Build history of the part. All positions in model axes, mm. Round coordinates to 2 decimals unless told otherwise and drop trailing zeros. Write each loop counter-clockwise with the first axis right and the second up, starting at its lowest first coordinate (ties: lowest second). Pieces come first, ordered by that corner, then holes.
Item 1: Band-saw the part on B-B, the plane z = -41.5. Write the cut outline in (x, y) (3 decimals), then the cut area to 3 significant figures.
Item 2: Band-saw the part on A-A, the plane y = 2.3. Write the cut outline in (x, z) (3 decimals).
Item 3: Band-saw the part on D-D, the plane x = 212.5. Write the cut outline in (y, z) (3 decimals), then the cut area to 3 significant figures.
Item 4: Wall check: probe 1 along Z at (x, y) = (272, 2.35); probe 2 along X at (y, z) = (0.55, -132); probe 3 along Z at (x, y) = (229, 2.55). Give the ranges that are in metal, low to high.
Item 5: Band-saw the part on C-C, the plane z = -135. Write the cut outline in (x, y) (3 decimals), then the cut area to 3 significant figures.
```python
from build123d import *

# Parameters (mm, degrees)
SKETCH1_W           = 679.45
SKETCH1_H           = 368.3
BOSS_EXTRUDE1_DEPTH = 3.175
CUT_EXTRUDE1_DEPTH  = 4.175


with BuildPart() as part:
    # Sketch1 → Boss-Extrude1 (new body)
    with BuildSketch(Plane(origin=(0, 0, 0), x_dir=(1, 0, 0), z_dir=(0, 1, 0))):
        with Locations((339.725, 184.15)):
            Rectangle(SKETCH1_W, SKETCH1_H)
    extrude(amount=BOSS_EXTRUDE1_DEPTH)

    # Sketch2 → Cut-Extrude1 (cut, through all)
    with BuildSketch(Plane(origin=(0, 3.175, 0), x_dir=(1, 0, 0), z_dir=(0, 1, 0))):
        with BuildLine():
            Line((135.832993334, 0), (144.943397545, 30.143073778))
            ThreePointArc((144.943397545, 30.143073778), (213.497085422, 129.330172419), (327.025, 169.939300333))
            ThreePointArc((327.025, 169.939300333), (472.568969877, 112.385716223), (530.122553987, -33.158253654))
            ThreePointArc((530.122553987, -33.158253654), (520.134888885, -89.022933623), (494.625079918, -139.71677515))
            add(Edge.make_bspline(
                [(494.625079918, -139.71677515), (493.45726691, -141.384584969), (490.895198527, -144.528294755), (484.77915912, -150.233837552), (475.335730084, -156.231610738), (461.521693133, -161.444305371), (379.648366594, -177.46097032), (267.722400389, -112.187788034), (488.667649379, 0)],
                knots=[0, 0, 0, 0, 0.027722316, 0.055444633, 0.110889265, 0.166333898, 0.22177853, 0.984715491, 0.984715491, 0.984715491, 0.984715491], degree=3))
            Line((488.667649379, 0), (135.832993334, 0))
        make_face()
    extrude(amount=-CUT_EXTRUDE1_DEPTH, mode=Mode.SUBTRACT)


solid = part.part
```
Results:
1. outline: (0, 0) - (148.757, 0) - (148.757, 3.175) - (0, 3.175) - close; (517.993, 0) - (679.45, 0) - (679.45, 3.175) - (517.993, 3.175) - close
1. area: 985 mm2
2. outline: (0, -368.3) - (679.45, -368.3) - (679.45, 0) - (528.391, 0) arc R196.85 cw to (144.943, -30.143) - (135.833, 0) - (0, 0) - close
3. outline: (0, -368.3) - (3.175, -368.3) - (3.175, -128.56) - (0, -128.56) - close
3. area: 761 mm2
4. probe 1: z = -368.3 to -160.23
4. probe 2: x = 0 to 217.06, 449.69 to 679.45
4. probe 3: z = -368.3 to -140.09
5. outline: (0, 0) - (221.268, 0) - (221.268, 3.175) - (0, 3.175) - close; (445.482, 0) - (679.45, 0) - (679.45, 3.175) - (445.482, 3.175) - close
5. area: 1,450 mm2
